For this review, take the finished solid that the model builds, in its own axes (mm). A direction names the side the tool comes from. Round coordinates to 2 decimals unless told otherwise and drop trailing zeros. Order: outer loops, then holes, each group sorted by start corner. A loop starts at its lowest first (then second) coordinate and runs counter-clockwise, first axis right, second up. Notation, with made-up numbers: (42, 33.5) -> (80, 33.5) arc R26 cw to (80, 50.5) -> close; hole circle Ø1 at (28.25, -32). An arc over 180 degrees is marked (long way). Answer in a Markdown table with one row per item.
```python
from build123d import *

# Parameters (mm, degrees)
SKETCH_1_W          = 130
SKETCH_1_H          = 290
EXTRUDE_1_DEPTH     = 3
SKETCH_3_W          = 30
SKETCH_3_H          = 34.54
CUT_EXTRUDE_3_DEPTH = 3
SKETCH_4_R          = 2
CUT_EXTRUDE_4_DEPTH = 3
CUT_EXTRUDE_6_DEPTH = 10
SKETCH_6_W          = 10
SKETCH_6_H          = 290
EXTRUDE_2_DEPTH     = 3
SKETCH_7_W          = 3
SKETCH_7_H          = 10
CUT_EXTRUDE_7_DEPTH = 6
SKETCH_8_W          = 3
SKETCH_8_H          = 10
CUT_EXTRUDE_8_DEPTH = 6


with BuildPart() as part:
    # 草图1 → 凸台-拉伸1 (new body)
    with BuildSketch(Plane(origin=(0, 0, 0), x_dir=(0, 0, -1), z_dir=(1, 0, 0))):
        with Locations((28.545134703, -106.027707237)):
            Rectangle(SKETCH_1_W, SKETCH_1_H)
    extrude(amount=EXTRUDE_1_DEPTH)

    # 草图3 → 切除-拉伸3 (cut)
    with BuildSketch(Plane(origin=(3, 0, 0), x_dir=(0, 0, -1), z_dir=(1, 0, 0))):
        with Locations((30.181306513, -28.135365108)):
            Rectangle(SKETCH_3_W, SKETCH_3_H)
    extrude(amount=-CUT_EXTRUDE_3_DEPTH, mode=Mode.SUBTRACT)

    # 草图4 → 切除-拉伸4 (cut)
    with BuildSketch(Plane(origin=(3, 0, 0), x_dir=(0, 0, -1), z_dir=(1, 0, 0))):
        with Locations((52.181306513, -25.865365108)):
            Circle(SKETCH_4_R)
        with Locations((8.181306513, -25.865365108)):
            Circle(SKETCH_4_R)
    extrude(amount=-CUT_EXTRUDE_4_DEPTH, mode=Mode.SUBTRACT)

    # 草图5 → 切除-拉伸6 (cut)
    with BuildSketch(Plane.ZY):
        Polygon((-73.995657993, -116.121202928), (-73.995657993, -150.753178318), (-39.363682603, -116.121202928), align=None)
        Polygon((-25.221546979, -116.121202928), (-73.995657993, -164.895313942), (-73.995657993, -184.694303815), (-5.422557106, -116.121202928), align=None)
        Polygon((8.719578518, -116.121202928), (-73.995657993, -198.836439439), (-73.995657993, -216.121202928), (26.004342007, -116.121202928), align=None)
        Polygon((26.004342007, -130.263338551), (-59.85352237, -216.121202928), (-42.882959621, -216.121202928), (26.004342007, -147.2339013), align=None)
        Polygon((26.004342007, -161.376036924), (-28.740823997, -216.121202928), (-8.941834124, -216.121202928), (26.004342007, -181.175026797), align=None)
        Polygon((26.004342007, -195.317162421), (5.2003015, -216.121202928), (26.004342007, -216.121202928), align=None)
    extrude(amount=-CUT_EXTRUDE_6_DEPTH, mode=Mode.SUBTRACT)

    # 草图6 → 凸台-拉伸2 (add)
    with BuildSketch(Plane(origin=(3, 0, 0), x_dir=(0, 0, -1), z_dir=(1, 0, 0))):
        with Locations((88.545134703, -106.027707237)):
            Rectangle(SKETCH_6_W, SKETCH_6_H)
    extrude(amount=EXTRUDE_2_DEPTH)

    # 草图7 → 切除-拉伸7 (cut)
    with BuildSketch(Plane(origin=(0, 38.972292763, 0), x_dir=(1, 0, 0), z_dir=(0, 1, 0))):
        with Locations((4.5, 88.545134703)):
            Rectangle(SKETCH_7_W, SKETCH_7_H)
    extrude(amount=-CUT_EXTRUDE_7_DEPTH, mode=Mode.SUBTRACT)

    # 草图8 → 切除-拉伸8 (cut)
    with BuildSketch(Plane.XZ.offset(251.027707237)):
        with Locations((4.5, -88.545134703)):
            Rectangle(SKETCH_8_W, SKETCH_8_H)
    extrude(amount=-CUT_EXTRUDE_8_DEPTH, mode=Mode.SUBTRACT)


solid = part.part
```
Q1. The part is to be moulded in two halves that separate along Z. For faces 1 (the face through (1.48, -133.68, -56.92)), 2 (the face through (3, -108, -93.545)), 3 (the face through (6, -104, -88)), say which applies: +Z half, -Z half, draft (parallel to the pull), parting line (faces both ways), or undercut.
Answer key:
| item | result |
|---|---|
| face 1 | undercut |
| face 2 | -Z half |
| face 3 | draft |
Q2. Take a section at C-C, the plane x = 1.55. Give the number of separate pieces and of enclosed holes in the cut face, then the cut area to 3 significant figures.
Answer key:
| item | result |
|---|---|
| separate pieces | 1 |
| enclosed holes | 9 |
| area | 30,900 mm^2 |
Q3. Take a section at D-D, the plane y = -138.5. Write out the cut boundary in (x, z).
Answer key:
| item | result |
|---|---|
| outline | (0, -93.55) -> (6, -93.55) -> (6, -83.55) -> (3, -83.55) -> (3, -74) -> (0, -74) -> close; (0, -61.74) -> (3, -61.74) -> (3, -47.6) -> (0, -47.6) -> close; (0, -27.8) -> (3, -27.8) -> (3, -13.66) -> (0, -13.66) -> close; (0, 3.63) -> (3, 3.63) -> (3, 17.77) -> (0, 17.77) -> close; (0, 26) -> (3, 26) -> (3, 36.45) -> (0, 36.45) -> close |
Q4. Clearance check with flat-ended pins moving along their axes: pin 1 Ø2 at (y, z) = (7.5, 6) entering from +X; pin 2 Ø1.5 at (x, z) = (5, -90.5) entering from -Y. State where each tip first meets the part, or that it passes through.
Answer key:
| item | result |
|---|---|
| pin 1 | stops at x = 3 |
| pin 2 | stops at y = -245.03 |
Q5. Take a section at B-B, the plane z = -22. Write out the cut boundary in (x, y).
Answer key:
| item | result |
|---|---|
| outline | (0, -251.03) -> (3, -251.03) -> (3, -216.12) -> (0, -216.12) -> close; (0, -209.38) -> (3, -209.38) -> (3, -195.24) -> (0, -195.24) -> close; (0, -178.27) -> (3, -178.27) -> (3, -164.13) -> (0, -164.13) -> close; (0, -146.84) -> (3, -146.84) -> (3, -132.7) -> (0, -132.7) -> close; (0, -116.12) -> (3, -116.12) -> (3, -45.41) -> (0, -45.41) -> close; (0, -10.87) -> (3, -10.87) -> (3, 38.97) -> (0, 38.97) -> close |
Q6. To check wall thickness, follow probe 1 along Y at (x, z) = (1.6, -53.5); probe 2 along Y at (x, z) = (2.6, -61.5); probe 3 along Z at (x, y) = (0.9, -174). State the ranges of each line that lie inside material, in increasing order.
Answer key:
| item | result |
|---|---|
| probe 1 | y = -251.03 to -216.12, -209.77 to -195.63, -178.34 to -164.2, -144.4 to -130.26, -116.12 to -27.37, -24.36 to 38.97 |
| probe 2 | y = -251.03 to -203.63, -186.34 to -172.2, -152.4 to -138.26, -116.12 to 38.97 |
| probe 3 | z = -93.55 to -74, -63.3 to -49.16, -31.87 to -17.73, -0.76 to 13.38, 26 to 36.45 |
Q7. Take a section at A-A, the plane y = -34. Write out the cut boundary in (x, z).
Answer key:
| item | result |
|---|---|
| outline | (0, -93.55) -> (6, -93.55) -> (6, -83.55) -> (3, -83.55) -> (3, -45.18) -> (0, -45.18) -> close; (0, -15.18) -> (3, -15.18) -> (3, 36.45) -> (0, 36.45) -> close |
Q8. Tool access review of faces 4 (the face through (1.48, -172.59, -16.32)), 5 (the face through (0, -104, -28)): name each direction out of +Z, -Z, +X, -X, +Y, -Y from which nothing blocks a thin tool from reaching the whole face with its end or side.
Answer key:
| item | result |
|---|---|
| face 4 | +X, -X |
| face 5 | +Z, -Z, -X, +Y, -Y |
